Source: CAD feature listing. Evaluate the final solid. Frame: model axes, mm. A direction names the side the tool comes from. Coordinates: 2 decimals unless noted, no trailing zeros. Order: outer loops, then holes, each group sorted by start corner. A loop starts at its lowest first (then second) coordinate and runs counter-clockwise, first axis right, second up.
Item 1: Section B-B on x = 14. Return the cut outline in (y, z) (1 decimal).
Item 2: Contact query for flat-ended pins moving along their axis: P1, Ø1, axis at x = 13.5, y = -1, coming from the +Z side; P2, Ø3, axis at x = 10, y = 0, coming from the -Z side; P3, Ø1.5, axis at y = -0.5, z = -2.5, coming from the +X side (3 decimals). Output: stop coordinate, or through.
Item 3: Reachability of faces 4 (the flat face through (7, 3.175, -1)), 5 (the flat face through (0, 0, -1.588)) from +Z, -Z, +X, -X, +Y, -Y: full face, straight path, thin tool, end or side. Return the list, or none.
Item 4: Ray query, line 1 (Y direction, x = 15, z = -1.3) (1 decimal); line 2 (Z direction, x = 14, y = 2); line 3 (X direction, y = 0.25, z = -1.4). Return the intervals inside material, ascending.
Item 5: Mould query, pull axis Y, two halves, no side actions, for faces 1 (the flat face through (9, 0, -1.588)), 2 (the flat face through (8, -3.175, -1)), 3 (the cylindrical face through (0.34, -1.55, -3.15)). Classes: released by +Y, released by -Y, zero draft, split by the parting line, or undercut.
from build123d import *

# Parameters (mm, degrees)
SKETCH1_R           = 1.5875
BOSS_EXTRUDE1_DEPTH = 1.5875
SKETCH2_R           = 3.175
SKETCH2_R_2         = 1.5875
BOSS_EXTRUDE2_DEPTH = 3.175


with BuildPart() as part:
    # Sketch1 → Boss-Extrude1 (new body)
    with BuildSketch(Plane.XY):
        with BuildLine():
            Line((0, 3.175), (15, 3.175))
            ThreePointArc((15, 3.175), (18.175, 0), (15, -3.175))
            Line((15, -3.175), (0, -3.175))
            ThreePointArc((0, -3.175), (-3.175, 0), (0, 3.175))
        make_face()
        with Locations((15, 0)):
            Circle(SKETCH1_R, mode=Mode.SUBTRACT)
    extrude(amount=-BOSS_EXTRUDE1_DEPTH)

    # Sketch2 → Boss-Extrude2 (add)
    with BuildSketch(Plane(origin=(0, 0, -1.5875), x_dir=(-1, 0, 0), z_dir=(0, 0, -1))):
        with Locations(Location((0, 0, 0), (0, 0, 90))):
            Circle(SKETCH2_R)
        Circle(SKETCH2_R_2, mode=Mode.SUBTRACT)
    extrude(amount=BOSS_EXTRUDE2_DEPTH)


solid = part.part
Answer list:
1. outline: (-3.2, -1.6) - (-1.2, -1.6) - (-1.2, 0) - (-3.2, 0) - close; (1.2, -1.6) - (3.2, -1.6) - (3.2, 0) - (1.2, 0) - close
2. P1: stops at z = 0
2. P2: stops at z = -1.59
2. P3: stops at x = 3.175
3. face 4: +Z, -Z, +X, -X, +Y
3. face 5: -Z
4. line 1: y = -3.2 to -1.6, 1.6 to 3.2
4. line 2: z = -1.59 to 0
4. line 3: x = -3.17 to 13.43, 16.57 to 18.17
5. face 1: zero draft
5. face 2: released by -Y
5. face 3: undercut
